Autodesk Inventor part; units mm, degrees
ref_plane "YZ Plane" through (0, 0, 0) normal (1, 0, 0) x (0, 1, 0)
ref_plane "XZ Plane" through (0, 0, 0) normal (0, 1, 0) x (-1, 0, 0)
ref_plane "XY Plane" through (0, 0, 0) normal (0, 0, 1) x (1, 0, 0)
sketch "Sketch1" plane through (0, 0, 0) normal (0, 1, 0) x (-1, 0, 0)
  line L0 (-33.5, 41.5) -> (33.5, 41.5)
  line L1 (33.5, 41.5) -> (33.5, -41.5)
  line L2 (33.5, -41.5) -> (-33.5, -41.5)
  line L3 (-33.5, -41.5) -> (-33.5, 41.5)
  line L4 (-33.5, 41.5) -> (33.5, -41.5) construction
  line L5 (33.5, 41.5) -> (-33.5, -41.5) construction
  point P0 (0, 0)
  dimension "d0" = 67
  dimension "d1" = 83
extrude "Extrusion1" add sketch "Sketch1" along normal blind 3
sketch "Sketch2" plane through (0, 3, 0) normal (0, 1, 0) x (1, 0, 0)
  line L0 (-33.5, 41.5) -> (-33.5, -41.5)
  line L1 (33.5, 41.5) -> (-33.5, 41.5)
  line L2 (-33.5, 41.5) -> (-33.5, -41.5)
  line L3 (-33.5, -41.5) -> (33.5, -41.5)
  line L4 (33.5, -41.5) -> (33.5, 41.5)
  line L5 (33.5, 41.5) -> (-33.5, -41.5) construction
  line L6 (-33.5, 41.5) -> (33.5, -41.5) construction
  line L7 (30.5, 38.5) -> (-30.5, 38.5)
  line L8 (-30.5, 38.5) -> (-30.5, -38.5)
  line L9 (-30.5, -38.5) -> (30.5, -38.5)
  line L10 (30.5, -38.5) -> (30.5, 38.5)
  line L11 (30.5, 38.5) -> (-30.5, -38.5) construction
  line L12 (-30.5, 38.5) -> (30.5, -38.5) construction
  point P0 (0, 0)
  dimension "d4" = 61
  dimension "d5" = 77
extrude "Extrusion2" add sketch "Sketch2" along normal blind 5
sketch "Sketch3" plane through (0, 3, 0) normal (0, 1, 0) x (1, 0, 0)
  circle A0 centre (21, 27) radius 1.75
  line L0 (-30.5, 38.5) -> (30.5, 38.5)
  line L1 (30.5, 38.5) -> (30.5, -38.5)
  circle A1 centre (21, -28) radius 1.75
  circle A2 centre (-17, 27) radius 1.75
  circle A3 centre (-17, -28) radius 1.75
  point P0 (0, 0)
  point P1 (30.5, -38.5)
  point P2 (26, 41.5)
  point P3 (26, -41.5)
  dimension "d8" = 3.5
  dimension "d9" = 11.5
  dimension "d10" = 9.5
  dimension "d13" = 55
  dimension "d16" = 38
extrude "Extrusion3" cut sketch "Sketch3" against normal blind 5
fillet "Fillet1" radius 4 4 edges at (33.5, 0, 0) (-33.5, 0, 0) (0, 0, 41.5) (0, 0, -41.5)
fillet "Fillet2" radius 2 4 edges at (-30.5, 5.5, -38.5) (30.5, 5.5, -38.5) (30.5, 5.5, 38.5) (-30.5, 5.5, 38.5)
properties part number "Motor_Node_top"
Geometry: final body of the model. Coordinates: model frame, mm. A direction names the side the tool comes from. Give positions to 0.01 mm unless a question says otherwise; leave off trailing zeros. Write each loop counter-clockwise with the first axis right and the second up, starting at its lowest first coordinate (ties: lowest second). Pieces come first, ordered by that corner, then holes. Notation, with made-up numbers: (-36.75, 2.25) - (-13.75, 2.25) arc R26 cw to (-13.75, 17.25) - close; hole circle Ø5 at (-15.5, -4). An arc over 180 degrees is marked (long way). Return JSON: item names as keys, results as strings. Group by question number.
1) Set-up query: faces 1 (the cylindrical face through (-18.29, 1.52, -28.18)), 2 (the flat face through (0, 3, 1)). Return all of +Z, -Z, +X, -X, +Y, -Y with unobstructed straight access to the full face (end or side cutting, diameter ignored); none if empty.
2) Line query: line 1 (Z direction, x = -4, y = 7.75); line 2 (Z direction, x = 21, y = 1.8); line 3 (X direction, y = 2, z = -27). Output: solid intervals per line, ascending.
3) First-contact query: P1, Ø4, axis at x = -12.5, y = 3.5, coming from the -Z side; P2, Ø10, axis at x = -21.5, z = 23.5, coming from the +Y side; P3, Ø1, axis at y = 2, z = 20, coming from the +X side; P4, Ø3, axis at y = 2, z = -20, coming from the +X side. Flat tips, straight axial feed; report the tip coordinate or a pass-through.
4) Section D-D on z = -0.5. Return the cut outline in (x, y), plus the area to 3 significant figures.
5) Section A-A on z = -27. Return the cut outline in (x, y).
6) Section C-C on y = 5.75. Return the cut outline in (x, z), plus the area to 3 significant figures.
7) Section B-B on x = -17. Return the cut outline in (y, z), plus the area to 3 significant figures.
Filled in:
{
 "1": {"face 1": "+Y, -Y", "face 2": "+Y"},
 "2": {"line 1": "z = -41.5 to -38.5, 38.5 to 41.5", "line 2": "z = -40.84 to -28.75, -25.25 to 26.25, 29.75 to 40.84", "line 3": "x = -32.96 to -18.75, -15.25 to 19.25, 22.75 to 32.96"},
 "3": {"P1": "stops at z = -41.5", "P2": "stops at y = 3", "P3": "stops at x = 33.21", "P4": "stops at x = 33.47"},
 "4": {"outline": "(-33.5, 4) arc R4 ccw to (-29.5, 0) - (29.5, 0) arc R4 ccw to (33.5, 4) - (33.5, 8) - (30.5, 8) - (30.5, 3) - (-30.5, 3) - (-30.5, 8) - (-33.5, 8) - close", "area": "224 mm^2"},
 "5": {"outline": "(-33.5, 4) arc R4 ccw to (-29.5, 0) - (-18.75, 0) - (-18.75, 3) - (-30.5, 3) - (-30.5, 8) - (-33.5, 8) - close; (-15.25, 0) - (19.25, 0) - (19.25, 3) - (-15.25, 3) - close; (22.75, 0) - (29.5, 0) arc R4 ccw to (33.5, 4) - (33.5, 8) - (30.5, 8) - (30.5, 3) - (22.75, 3) - close"},
 "6": {"outline": "(-33.5, -41.5) - (33.5, -41.5) - (33.5, 41.5) - (-33.5, 41.5) - close; hole (-30.5, -36.5) arc R2 ccw to (-28.5, -38.5) - (28.5, -38.5) arc R2 ccw to (30.5, -36.5) - (30.5, 36.5) arc R2 ccw to (28.5, 38.5) - (-28.5, 38.5) arc R2 ccw to (-30.5, 36.5) - close", "area": "867 mm^2"},
 "7": {"outline": "(0, -37.5) arc R4 ccw to (4, -41.5) - (8, -41.5) - (8, -38.5) - (3, -38.5) - (3, -28.75) - (0, -28.75) - close; (0, -25.25) - (3, -25.25) - (3, 26.25) - (0, 26.25) - close; (0, 29.75) - (3, 29.75) - (3, 38.5) - (8, 38.5) - (8, 41.5) - (4, 41.5) arc R4 ccw to (0, 37.5) - close", "area": "251 mm^2"}
}
